```python
from build123d import *

# Parameters (mm, degrees)
F1_DEPTH = 63.5
F3_DEPTH = 38.1
F2_R     = 12.7
F4_DEPTH = 38.1
F5_DEPTH = 273.05


with BuildPart() as f1:
    # F0 (on Front) → F1 (new body, symmetric)
    with BuildSketch(Plane.XZ):
        Polygon((0, 87.400968), (0, 0), (304.8, 0), (304.8, 101.6), (266.7, 101.6), (266.7, 38.1), (31.75, 38.1), (31.75, 101.6), (12.7, 101.6), align=None)
    extrude(amount=F1_DEPTH, both=True)

    # F2 (on face) → F3 (cut)
    with BuildSketch(Plane.YZ.offset(304.8)):
        with BuildLine():
            Line((-63.5, 101.6), (-63.5, 50.8))
            Line((-63.5, 50.8), (-47.160853, 50.8))
            Line((-47.160853, 50.8), (-21.208122, 90.177681))
            ThreePointArc((-21.208122, 90.177681), (-12.044229, 98.562839), (0, 101.6))
            Line((0, 101.6), (-63.5, 101.6))
        make_face()
        with BuildLine():
            Line((63.5, 101.6), (0, 101.6))
            ThreePointArc((0, 101.6), (11.862834, 98.65959), (20.979086, 90.519147))
            Line((20.979086, 90.519147), (48.089147, 50.8))
            Line((48.089147, 50.8), (63.5, 50.8))
            Line((63.5, 50.8), (63.5, 101.6))
        make_face()
    extrude(amount=-F3_DEPTH, mode=Mode.SUBTRACT)

    # F2 (on face) → F4 (cut)
    with BuildSketch(Plane.YZ.offset(304.8)):
        with Locations((0, 76.2)):
            Circle(F2_R)
    extrude(amount=-F4_DEPTH, mode=Mode.SUBTRACT)

    # F2 (on face) → F5 (cut)
    with BuildSketch(Plane.YZ.offset(304.8)):
        Polygon((-12.7, 16.51), (-12.7, 0), (12.7, 0), (12.7, 16.51), (31.75, 16.51), (31.75, 29.21), (12.7, 29.21), (12.7, 38.1), (-12.7, 38.1), (-12.7, 29.21), (-31.75, 29.21), (-31.75, 16.51), align=None)
    extrude(amount=-F5_DEPTH, mode=Mode.SUBTRACT)


solid = f1.part
```
The listing builds one solid part. Answer for the finished solid, in the listing's coordinates (mm). A direction names the side the tool comes from. Round coordinates to 2 decimals unless told otherwise and drop trailing zeros. Loops run counter-clockwise (first coordinate to the right, second up) from the corner with the lowest first, then second, coordinate; pieces in that order, holes last.
Q1. Find the intervals of material crossed by line 1 (Z direction, x = 275, y = 0); line 2 (X direction, y = -21, z = 63.5); line 3 (Z direction, x = 177, y = -22), in increasing order.
Q2. Section D-D, the plane y = -50 is taken. Determine the outline of the cut face in (x, z), then the cut area to 3 significant figures.
Q3. For a pull along Y with two mould halves and no side action, classify faces 6 (the face through (170, -31.75, 23)), 7 (the face through (304.8, -1, 39)), 8 (the face through (116, 63.5, 29)) as released by +Y, released by -Y, zero draft, split by the parting line, or undercut.
Q4. Section A-A, the plane y = -9.5 is taken. Determine the outline of the cut face in (x, z).
Q5. Which of the six approach directions +Z, -Z, +X, -X, +Y, -Y give full straight-line access (tool end or side, diameter ignored) to faces 1 (the face through (170, -22, 29.21)), 2 (the face through (286, 0, 38.1)), 3 (the face through (0, -1, 44)), 4 (the face through (286.017, 34.344, 70.938)), 5 (the face through (151, -38, 38.1))?
Q6. Section B-B, the plane x = 89 is taken. Determine the outline of the cut face in (y, z), then the cut area to 3 significant figures.
Q7. Section C-C, the plane z = 76.2 is taken. Determine the outline of the cut face in (x, y), then the cut area to 3 significant figures.
Q8. Given pin 1 Ø10 at (y, z) = (-38, 70.5) entering from +X; pin 2 Ø18 at (x, y) = (288, -58.5) entering from +Z; pin 3 Ø15 at (x, y) = (199, 25) entering from +Z, each flat-ended and moving along its own axis, determine where each tip first touches the part or whether it passes through.
Completed:
1. line 1: z = 38.1 to 63.5, 88.9 to 101.6
1. line 2: x = 0 to 31.75, 266.7 to 304.8
1. line 3: z = 0 to 16.51, 29.21 to 38.1
2. outline: (0, 0) - (304.8, 0) - (304.8, 50.8) - (266.7, 50.8) - (266.7, 38.1) - (31.75, 38.1) - (31.75, 101.6) - (12.7, 101.6) - (0, 87.4) - close
2. area: 14,000 mm2
3. face 6: undercut
3. face 7: zero draft
3. face 8: released by +Y
4. outline: (0, 0) - (31.75, 0) - (31.75, 101.6) - (12.7, 101.6) - (0, 87.4) - close; (266.7, 38.1) - (304.8, 38.1) - (304.8, 67.77) - (266.7, 67.77) - close; (266.7, 84.63) - (304.8, 84.63) - (304.8, 99.76) - (266.7, 99.76) - close
5. face 1: +X
5. face 2: -Z, +X
5. face 3: +Z, -Z, -X, +Y, -Y
5. face 4: +Z, +X, +Y
5. face 5: +Z, +Y, -Y
6. outline: (-63.5, 0) - (-12.7, 0) - (-12.7, 16.51) - (-31.75, 16.51) - (-31.75, 29.21) - (-12.7, 29.21) - (-12.7, 38.1) - (-63.5, 38.1) - close; (12.7, 0) - (63.5, 0) - (63.5, 38.1) - (12.7, 38.1) - (12.7, 29.21) - (31.75, 29.21) - (31.75, 16.51) - (12.7, 16.51) - close
6. area: 3,390 mm2
7. outline: (0, -63.5) - (31.75, -63.5) - (31.75, 63.5) - (0, 63.5) - close; (266.7, -30.42) - (304.8, -30.42) - (304.8, -12.7) - (266.7, -12.7) - close; (266.7, 12.7) - (304.8, 12.7) - (304.8, 30.75) - (266.7, 30.75) - close
7. area: 5,400 mm2
8. pin 1: stops at x = 304.8
8. pin 2: stops at z = 50.8
8. pin 3: stops at z = 38.1
